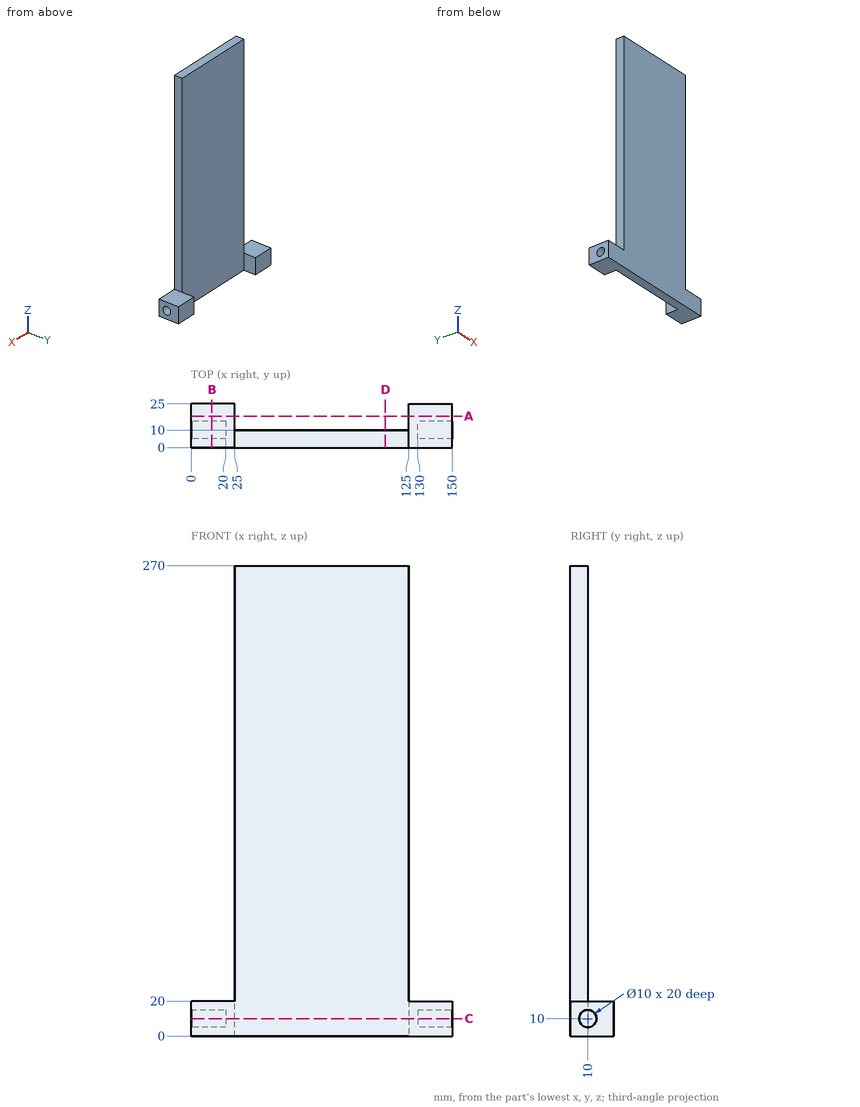
Design review of the part shown in the three views and the two pictorial views. Dimensions are in mm from the part's minimum x, y and z. Round coordinates to 2 decimals unless told otherwise and drop trailing zeros. Write each loop counter-clockwise with the first axis right and the second up, starting at its lowest first coordinate (ties: lowest second). Pieces come first, ordered by that corner, then holes.
1) Take a section at D-D on x = 111.5. Give the boundary of the cut face in (y, z), then the cut area to 3 significant figures.
Answer below:
outline: (0, 0) - (10, 0) - (10, 270) - (0, 270) - close
area: 2,700 mm2
2) Take a section at A-A on y = 18. Give the boundary of the cut face in (x, z).
Answer below:
outline: (0, 0) - (25, 0) - (25, 20) - (0, 20) - close; (125, 0) - (150, 0) - (150, 20) - (125, 20) - close
3) Insertion check: pin 1 Ø8 at (y, z) = (4.5, 166.5) entering from -X; pin 2 Ø6 at (y, z) = (10, 10) entering from +X; pin 3 Ø3 at (y, z) = (7.5, 9) entering from -X. Each pin has a flat end and moves straight along its axis. Give the tip position at first contact, or say it passes through.
Answer below:
pin 1: stops at x = 25
pin 2: stops at x = 130
pin 3: stops at x = 20
4) For line 1 along Y through (x, z) = (140, 10); line 2 along Z through (x, y) = (140.75, 10); line 3 along X through (y, z) = (8.5, 168), list the stretches that pass through material, from the lowest coordinate up.
Answer below:
line 1: y = 0 to 5, 15 to 25
line 2: z = 0 to 5, 15 to 20
line 3: x = 25 to 125
5) Take a section at C-C on z = 10. Give the boundary of the cut face in (x, y), then the cut area to 3 significant figures.
Answer below:
outline: (0, 0) - (150, 0) - (150, 5) - (130, 5) - (130, 15) - (150, 15) - (150, 25) - (125, 25) - (125, 10) - (25, 10) - (25, 25) - (0, 25) - (0, 15) - (20, 15) - (20, 5) - (0, 5) - close
area: 1,850 mm2
6) Take a section at B-B on x = 12. Give the boundary of the cut face in (y, z).
Answer below:
outline: (0, 0) - (25, 0) - (25, 20) - (0, 20) - close; hole circle Ø10 at (10, 10)
